Input: dimensioned drawing with shaded views. Units: mm. Origin: part minimum x, y, z. Round coordinates to 2 decimals unless told otherwise and drop trailing zeros. Loops run counter-clockwise (first coordinate to the right, second up) from the corner with the lowest first, then second, coordinate; pieces in that order, holes last. Notation, with made-up numbers: M 23,-5.75 L 52,-5.75 A30 cw 52,31.25 Z; hole C 34.5,67.25 d2. An arc over 180 degrees is marked long. Return JSON: item names as keys, results as strings.
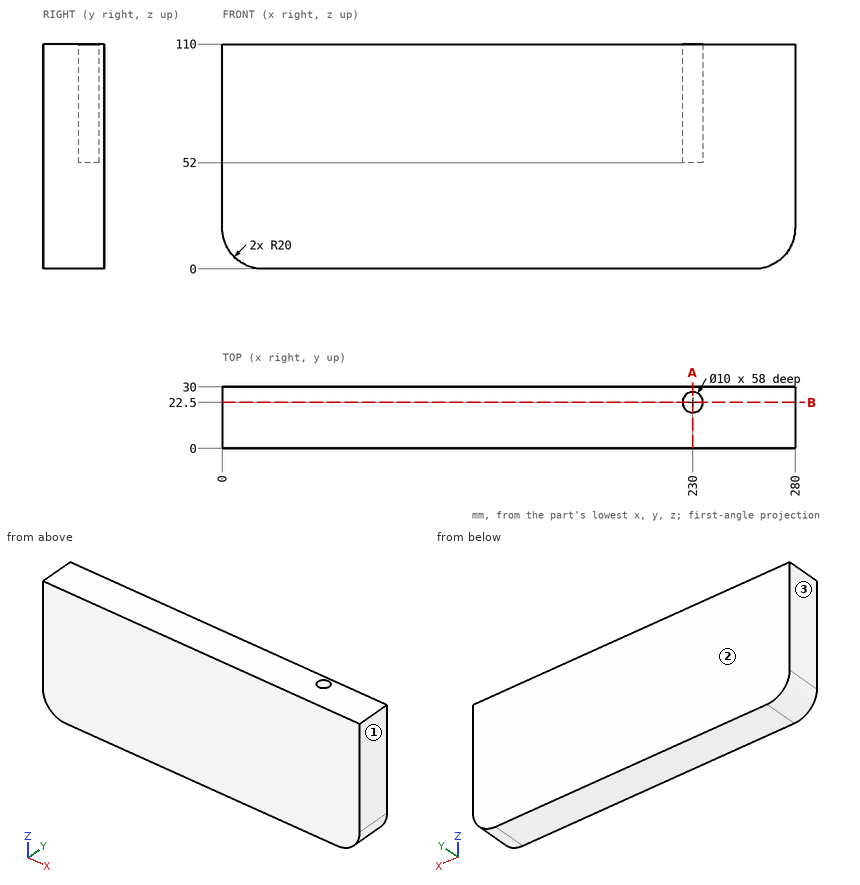
Q1. Section query A-A (x = 230). Output: boundary loops of the cut face in (y, z), plus the area to 3 significant figures.
Determined:
{"outline": "M 0,0 L 30,0 L 30,110 L 27.5,110 L 27.5,52 L 17.5,52 L 17.5,110 L 0,110 Z", "area": "2,720 mm^2"}
Q2. Pin query (flat end, axial travel): pin 1 (9 mm diameter, centred on x = 230, y = 22.5, fed in from +Z). Return the tip coordinate at first contact, or that it passes through.
Determined:
{"pin 1": "stops at z = 52"}
Q3. Material intervals for L1, parallel to Y at x = 230, z = 87; L2, parallel to X at y = 23.75, z = 88; L3, parallel to X at y = 2, z = 11, sorted ascending.
Determined:
{"L1": "y = 0 to 17.5, 27.5 to 30", "L2": "x = 0 to 225.16, 234.84 to 280", "L3": "x = 2.14 to 277.86"}
Q4. Pull-direction query (X, two-part tool) for the marked faces 1, 2 and 3; classes: pulls with the +X half, pulls with the -X half, needs draft (parallel to the pull), parting line crosses it, or undercut.
Determined:
{"face 1": "pulls with the +X half", "face 2": "needs draft", "face 3": "pulls with the -X half"}
Q5. Section query B-B (y = 22.5). Output: boundary loops of the cut face in (x, z).
Determined:
{"outline": "M 0,20 A20 ccw 20,0 L 260,0 A20 ccw 280,20 L 280,110 L 235,110 L 235,52 L 225,52 L 225,110 L 0,110 Z"}
